Build history of the part. All positions in model axes, mm. Round coordinates to 2 decimals unless told otherwise and drop trailing zeros. Loops run counter-clockwise (first coordinate to the right, second up) from the corner with the lowest first, then second, coordinate; pieces in that order, holes last. Notation, with made-up numbers: (-22, 3) - (23, 3) arc R13 cw to (23, 8) - close; hole circle Ø1 at (34, 50). An arc over 180 degrees is marked (long way). Use a Markdown table: item, result.
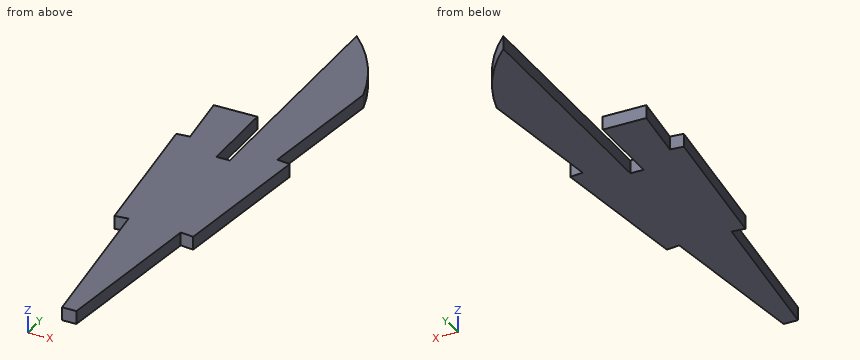
from build123d import *

# Parameters (mm, degrees)
BOSS_EXTRUDE1_DEPTH = 1.524
SKETCH2_W           = 10.339952981
SKETCH2_H           = 21.008044078
CUT_EXTRUDE1_DEPTH  = 1.524


with BuildPart() as part:
    # Sketch1 → Boss-Extrude1 (new body)
    with BuildSketch(Plane.XY):
        with BuildLine():
            Line((0, -185.062075144), (-1.524, -185.062075144))
            Line((-1.524, -185.062075144), (-1.524, -157.15233073))
            ThreePointArc((-1.524, -157.15233073), (-5.202982181, -161.792523258), (-7.537553978, -167.234588225))
            Line((-7.537553978, -167.234588225), (-5.752935589, -182.708365208))
            Line((-5.752935589, -182.708365208), (-7.266899912, -182.882973423))
            Line((-7.266899912, -182.882973423), (-5.263633807, -200.252565221))
            Line((-5.263633807, -200.252565221), (-3.749669484, -200.077957006))
            Line((-3.749669484, -200.077957006), (-1.585117021, -218.846004156))
            Line((-1.585117021, -218.846004156), (0.061117021, -218.846004156))
            Line((0.061117021, -218.846004156), (2.225669484, -200.077957006))
            Line((2.225669484, -200.077957006), (3.739633807, -200.252565221))
            Line((3.739633807, -200.252565221), (5.742899912, -182.882973423))
            Line((5.742899912, -182.882973423), (4.228935589, -182.708365208))
            Line((4.228935589, -182.708365208), (6.013553978, -167.234588225))
            ThreePointArc((6.013553978, -167.234588225), (3.678982181, -161.792523258), (0, -157.15233073))
            Line((0, -157.15233073), (0, -185.062075144))
        make_face()
    extrude(amount=BOSS_EXTRUDE1_DEPTH)

    # Sketch2 → Cut-Extrude1 (cut)
    with BuildSketch(Plane.XY.offset(1.524)):
        with Locations((-6.693976491, -165.555147297)):
            Rectangle(SKETCH2_W, SKETCH2_H)
    extrude(amount=-CUT_EXTRUDE1_DEPTH, mode=Mode.SUBTRACT)


solid = part.part
Q1. Cut at B-B, the plane y = -177. List the corners of the cut face in (x, z).
Results found:
| item | result |
|---|---|
| outline | (-6.41, 0) - (-1.52, 0) - (-1.52, 1.52) - (-6.41, 1.52) - close; (0, 0) - (4.89, 0) - (4.89, 1.52) - (0, 1.52) - close |
Q2. Drop flat-ended pins along their axis: pin 1 (0.5 mm diameter, centred on x = -1, z = 1, fed in from +Y); pin 2 (0.5 mm diameter, centred on y = -174.5, z = 1, fed in from -X). Give the stop position or say it passes through.
Results found:
| item | result |
|---|---|
| pin 1 | stops at y = -185.06 |
| pin 2 | stops at x = 0 |
Q3. Cut at C-C, the plane x = -1. List the corners of the cut face in (y, z), plus the area to 3 significant figures.
Results found:
| item | result |
|---|---|
| outline | (-218.85, 0) - (-185.06, 0) - (-185.06, 1.52) - (-218.85, 1.52) - close |
| area | 51.5 mm2 |
Q4. Cut at A-A, the plane z = 0.75. List the corners of the cut face in (x, y), plus the area to 3 significant figures.
Results found:
| item | result |
|---|---|
| outline | (-7.27, -182.88) - (-5.26, -200.25) - (-3.75, -200.08) - (-1.59, -218.85) - (0.06, -218.85) - (2.23, -200.08) - (3.74, -200.25) - (5.74, -182.88) - (4.23, -182.71) - (6.01, -167.23) arc R22.4 ccw to (0, -157.15) - (0, -185.06) - (-1.52, -185.06) - (-1.52, -176.06) - (-6.52, -176.06) - (-5.75, -182.71) - close |
| area | 406 mm2 |
Q5. Cut at D-D, the plane y = -208. List the corners of the cut face in (x, z), plus the area to 3 significant figures.
Results found:
| item | result |
|---|---|
| outline | (-2.84, 0) - (1.31, 0) - (1.31, 1.52) - (-2.84, 1.52) - close |
| area | 6.32 mm2 |
Q6. Probe line 1 (Y direction, x = -1.25, z = 1.2); line 2 (X direction, y = -179.5, z = 0.65); line 3 (X direction, y = -181, z = 1.3). List the from-to ranges inside material, lowest first.
Results found:
| item | result |
|---|---|
| line 1 | y = -218.85 to -185.06 |
| line 2 | x = -6.12 to -1.52, 0 to 4.6 |
| line 3 | x = -5.95 to -1.52, 0 to 4.43 |
